from build123d import *

# Parameters (mm, degrees)
SKETCH1_W               = 10
SKETCH1_H               = 5
BOSS_EXTRUDE1_DEPTH     = 300
CUT_EXTRUDE2_DEPTH      = 301.20217644
CUT_EXTRUDE2_DEPTH_BACK = 301.20217644
SKETCH3_R               = 1.5


with BuildPart() as part:
    # Sketch1 → Boss-Extrude1 (new body)
    with BuildSketch(Plane.XY):
        with Locations((0.232067511, -2.120253165)):
            Rectangle(SKETCH1_W, SKETCH1_H)
    extrude(amount=BOSS_EXTRUDE1_DEPTH)

    # Sketch3 → Cut-Extrude2 (cut, two sides: drawn at the far end of the back side and taken through both)
    with BuildSketch(Plane.ZY.offset(4.767932489).offset(-CUT_EXTRUDE2_DEPTH_BACK)):
        with Locations(Location((250, -2.120253165, 0), (0, 0, 270))):
            Circle(SKETCH3_R)
        with Locations(Location((50, -2.120253165, 0), (0, 0, 270))):
            Circle(SKETCH3_R)
    extrude(amount=CUT_EXTRUDE2_DEPTH + CUT_EXTRUDE2_DEPTH_BACK, mode=Mode.SUBTRACT)


solid = part.part
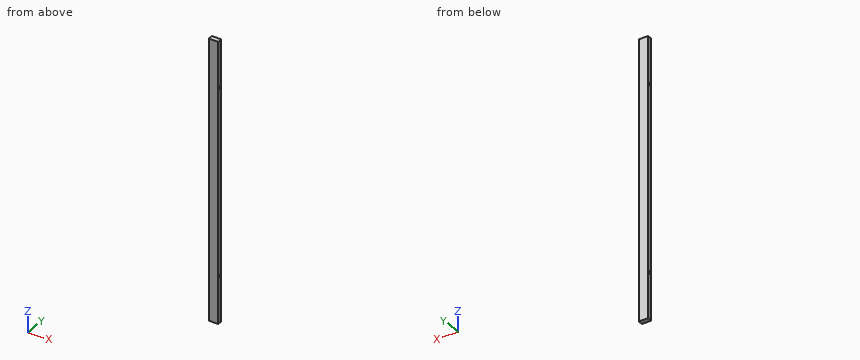
The model under review builds one solid part; all positions refer to its coordinate system, in mm. Round coordinates to 2 decimals unless told otherwise and drop trailing zeros. Order: outer loops, then holes, each group sorted by start corner. A loop starts at its lowest first (then second) coordinate and runs counter-clockwise, first axis right, second up. Notation, with made-up numbers: (19.5, 75.25) -> (26.5, 75.25) arc R33 ccw to (26.5, 106.25) -> close; hole circle Ø7 at (62.25, 69.25). An arc over 180 degrees is marked (long way). Use CSV: the item, a comma, the result in double quotes. Start each with the question number.
(1) Consider section A-A on y = -1.7. Write out the cut boundary in (x, z).
(2) Wall thickness on probe 1 along Z at (x, y) = (0.75, -1.8); probe 2 along Y at (x, z) = (1, 50); probe 3 along Z at (x, y) = (-3.75, -3.25): over which ranges is each line inside the solid? List them lowest first. Write a range as from..to.
(3) Insertion check: pin 1 (2.5 mm diameter, centred on y = -2.12, z = 250, fed in from +X). The pin has a flat end and moves straight along its axis. Give the tip position at first contact, or say it passes through.
Responses:
1,outline,"(-4.77, 0) -> (5.23, 0) -> (5.23, 48.56) -> (-4.77, 48.56) -> close; (-4.77, 51.44) -> (5.23, 51.44) -> (5.23, 248.56) -> (-4.77, 248.56) -> close; (-4.77, 251.44) -> (5.23, 251.44) -> (5.23, 300) -> (-4.77, 300) -> close"
2,probe 1,"0..48.53, 51.47..248.53, 251.47..300"
2,probe 2,"-4.62..-3.62, -0.62..0.38"
2,probe 3,"0..49.01, 50.99..249.01, 250.99..300"
3,pin 1,"through"
